Geometry check sheet. Reference: the model listing, model coordinates, mm. A direction names the side the tool comes from. Coordinates: 2 decimals unless noted, no trailing zeros. Write each loop counter-clockwise with the first axis right and the second up, starting at its lowest first coordinate (ties: lowest second). Pieces come first, ordered by that corner, then holes. Notation, with made-up numbers: (-7.5, 17.25) -> (13.5, 17.25) arc R11 ccw to (13.5, 24.25) -> close; hole circle Ø2 at (31, 4.25). An arc over 180 degrees is marked (long way). Answer in a Markdown table with one row per item. Add a question column.
Q1. Thickness scan on line 1 (Z direction, x = 3, y = 1); line 2 (Z direction, x = 4.25, y = -2); line 3 (X direction, y = -0.25, z = 60). Record the ranges inside material, lowest first.
Q2. Gauge pin test, flat ends, axial feed: P1, Ø1.5, axis at x = -3, y = -3, coming from the -Z side; P2, Ø5, axis at x = -3.5, z = 42.5, coming from the -Y side; P3, Ø2, axis at x = 3, z = 41.5, coming from the +Y side. Record the tip position at first contact, or that the pin passes through.
Q3. Section check A-A, the plane y = 0. Record the boundary of the cut face in (x, z).
Q4. Section check C-C, the plane z = -11. Record the boundary of the cut face in (x, y), and give its area (3 significant figures).
Q5. Section check D-D, the plane z = 30.5. Record the boundary of the cut face in (x, y), and give its area (3 significant figures).
Q6. Tool access check on faces 1 (the face through (0, 0, -16.176)), 2 (the face through (0, -3, -6)), 3 (the face through (-3.905, -0.867, 53.684)). Record the directions out of +Z, -Z, +X, -X, +Y, -Y that give a thin tool (end or side, any length) a straight path to the whole face; none if there is none.
Autodesk Inventor part; units mm, degrees
ref_plane "YZ Plane" through (0, 0, 0) normal (1, 0, 0) x (0, 1, 0)
ref_plane "XZ Plane" through (0, 0, 0) normal (0, 1, 0) x (-1, 0, 0)
ref_plane "XY Plane" through (0, 0, 0) normal (0, 0, 1) x (1, 0, 0)
sketch "Sketch1" plane through (0, 0, 0) normal (1, 0, 0) x (0, 1, 0)
  line L0 (0, -32.1759) -> (0, 79.8241) construction
  line L1 (0, 63.8241) -> (4, 63.8241)
  line L2 (4, 63.8241) -> (4, 43.8241)
  line L3 (4, 43.8241) -> (5, 43.8241)
  line L4 (5, 43.8241) -> (5, 23.8241)
  line L5 (5, 23.8241) -> (4, 23.8241)
  line L6 (4, 23.8241) -> (4, 3.8241)
  line L7 (4, 3.8241) -> (3, 3.8241)
  line L8 (3, 3.8241) -> (3, -16.1759)
  line L9 (3, -16.1759) -> (0, -16.1759)
  line L10 (0, 63.8241) -> (0, -16.1759)
  point P0 (0, 0)
  dimension "d0" = 3
  dimension "d1" = 80
  dimension "d2" = 60
  dimension "d3" = 20
  dimension "d4" = 4
  dimension "d5" = 5
revolve "Revolution1" add sketch "Sketch1" angle 360 about axis through (0, 0, 63.8241) along (0, 0, -1)
properties part number "02_Truc_01"
Calculated:
| question | item | result |
|---|---|---|
| 1 | line 1 | z = 3.82 to 63.82 |
| 1 | line 2 | z = 23.82 to 43.82 |
| 1 | line 3 | x = -3.99 to 3.99 |
| 2 | P1 | stops at z = 3.82 |
| 2 | P2 | stops at y = -4.9 |
| 2 | P3 | stops at y = 4.58 |
| 3 | outline | (-5, 23.82) -> (-4, 23.82) -> (-4, 3.82) -> (-3, 3.82) -> (-3, -16.18) -> (3, -16.18) -> (3, 3.82) -> (4, 3.82) -> (4, 23.82) -> (5, 23.82) -> (5, 43.82) -> (4, 43.82) -> (4, 63.82) -> (-4, 63.82) -> (-4, 43.82) -> (-5, 43.82) -> close |
| 4 | outline | circle Ø6 at (0, 0) |
| 4 | area | 28.3 mm² |
| 5 | outline | circle Ø10 at (0, 0) |
| 5 | area | 78.5 mm² |
| 6 | face 1 | -Z, +X, -X, +Y, -Y |
| 6 | face 2 | -Z |
| 6 | face 3 | +Z |
